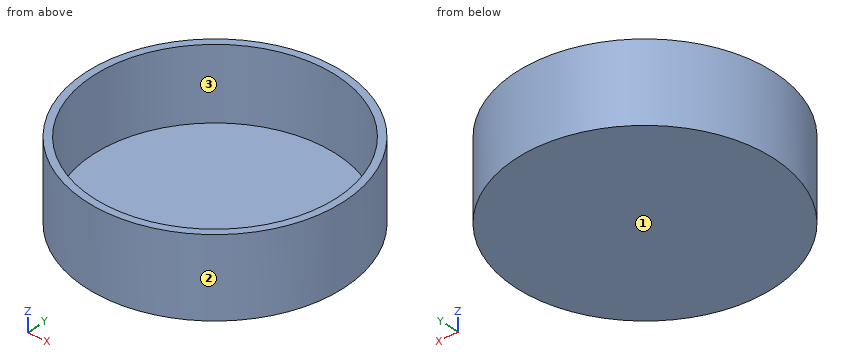
from build123d import *

# Parameters (mm, degrees)
SKETCH020_R  = 17
PAD018_DEPTH = 11
SKETCH019_R  = 18
PAD017_DEPTH = 11


with BuildPart() as body019:
    # Sketch020 → Pad018 (new body)
    with BuildSketch(Plane.XY.offset(-49)):
        with Locations((0, -37)):
            Circle(SKETCH020_R)
    extrude(amount=PAD018_DEPTH)


with BuildPart() as body019_1:
    # Body019 placement: moved
    add(body019.part.moved(Location((0, 0, 1))))


with BuildPart() as petri:
    # Sketch019 → Pad017 (new body)
    with BuildSketch(Plane.XY.offset(-49)):
        with Locations((0, -37)):
            Circle(SKETCH019_R)
    extrude(amount=PAD017_DEPTH)

    # Cut012: cut Body019
    add(body019_1.part, mode=Mode.SUBTRACT)


with BuildPart() as petri_1:
    # Cut012 placement: moved
    add(petri.part.moved(Location((0, 0, -12))))


solid = petri_1.part
Check sheet for the modelled part. Datum: model origin and axes. Units: mm. Face numbers are marked on the shaded views. Round coordinates to 2 decimals unless told otherwise and drop trailing zeros. Loops run counter-clockwise (first coordinate to the right, second up) from the corner with the lowest first, then second, coordinate; pieces in that order, holes last.
1. Scan lines: probe 1 along Y at (x, z) = (0, -52.75); probe 2 along Z at (x, y) = (7, -51.5); probe 3 along X at (y, z) = (-37.5, -51.5). Record each from-to range of solid material in increasing order.
2. Sectioned sample at B-B on x = 0. Record the boundary of the cut face in (y, z), and give its area (3 significant figures).
3. Mould release check, pull along X, two halves, no side actions. Record for the marked faces 1, 2 and 3: released by +X, released by -X, zero draft, split by the parting line, or undercut.
4. Gauge pin test, flat ends, axial feed: pin 1 Ø2 at (x, z) = (1.5, -54.5) entering from -Y; pin 2 Ø3 at (x, z) = (10.5, -55) entering from +Y; pin 3 Ø1.5 at (x, y) = (-11.5, -27.5) entering from +Z. Record the tip position at first contact, or that the pin passes through.
5. Sectioned sample at C-C on z = -59. Record the boundary of the cut face in (x, y).
6. Sectioned sample at A-A on y = -37. Record the boundary of the cut face in (x, z).
Recorded:
1. probe 1: y = -55 to -54, -20 to -19
1. probe 2: z = -61 to -60
1. probe 3: x = -17.99 to -16.99, 16.99 to 17.99
2. outline: (-55, -61) - (-19, -61) - (-19, -50) - (-20, -50) - (-20, -60) - (-54, -60) - (-54, -50) - (-55, -50) - close
2. area: 56.0 mm2
3. face 1: zero draft
3. face 2: split by the parting line
3. face 3: undercut
4. pin 1: stops at y = -54.99
4. pin 2: stops at y = -21.41
4. pin 3: stops at z = -60
5. outline: circle Ø36 at (0, -37); hole circle Ø34 at (0, -37)
6. outline: (-18, -61) - (18, -61) - (18, -50) - (17, -50) - (17, -60) - (-17, -60) - (-17, -50) - (-18, -50) - close
